```python
from build123d import *

# Parameters (mm, degrees)
SKETCH1_R           = 6.5
BOSS_EXTRUDE1_DEPTH = 1.5
SKETCH2_R           = 5.8
BOSS_EXTRUDE2_DEPTH = 4.3
FILLET1_R           = 0.4
SKETCH3_R           = 5
CUT_EXTRUDE1_DEPTH  = 4.8
BOSS_EXTRUDE3_DEPTH = 4.8
SKETCH5_W           = 2
SKETCH5_H           = 0.8
SKETCH5_W_2         = 1
SKETCH5_H_2         = 3.8
BOSS_EXTRUDE4_DEPTH = 7.2
CUT_EXTRUDE2_REACH  = 10.4
BOSS_EXTRUDE5_DEPTH = 3.8
FILLET2_R           = 0.1
FILLET3_R           = 0.2


with BuildPart() as part:
    # Sketch1 → Boss-Extrude1 (new body)
    with BuildSketch(Plane(origin=(0, 0, 0), x_dir=(1, 0, 0), z_dir=(0, 1, 0))):
        Circle(SKETCH1_R)
    extrude(amount=BOSS_EXTRUDE1_DEPTH)

    # Sketch2 → Boss-Extrude2 (add)
    with BuildSketch(Plane(origin=(0, 1.5, 0), x_dir=(1, 0, 0), z_dir=(0, 1, 0))):
        Circle(SKETCH2_R)
    extrude(amount=BOSS_EXTRUDE2_DEPTH)

    # Fillet1
    fillet1_edges = [part.edges().sort_by_distance(p)[0] for p in [
        (-5.8, 5.8, 0),
    ]]
    fillet(fillet1_edges, radius=FILLET1_R)

    # Sketch3 → Cut-Extrude1 (cut)
    with BuildSketch(Plane.XZ):
        Circle(SKETCH3_R)
    extrude(amount=-CUT_EXTRUDE1_DEPTH, mode=Mode.SUBTRACT)

    # Sketch4 → Boss-Extrude3 (add)
    with BuildSketch(Plane.XZ.offset(-4.8)):
        with BuildLine():
            Line((-4.990991885, 0.3), (-2.9, 0.3))
            Line((-2.9, 0.3), (-2.9, -0.3))
            Line((-2.9, -0.3), (-4.990991885, -0.3))
            ThreePointArc((-4.990991885, -0.3), (-5, 0), (-4.990991885, 0.3))
        make_face()
        with BuildLine():
            Line((2.9, 0.3), (2.9, -0.3))
            Line((2.9, -0.3), (4.990991885, -0.3))
            ThreePointArc((4.990991885, -0.3), (5, 0), (4.990991885, 0.3))
            Line((4.990991885, 0.3), (2.9, 0.3))
        make_face()
        with BuildLine():
            Line((-0.3, 4.990991885), (-0.3, 2.7))
            Line((-0.3, 2.7), (0.3, 2.7))
            Line((0.3, 2.7), (0.3, 4.990991885))
            ThreePointArc((0.3, 4.990991885), (0, 5), (-0.3, 4.990991885))
        make_face()
        with BuildLine():
            Line((0.3, -2.7), (-0.3, -2.7))
            Line((-0.3, -2.7), (-0.3, -4.990991885))
            ThreePointArc((-0.3, -4.990991885), (0, -5), (0.3, -4.990991885))
            Line((0.3, -4.990991885), (0.3, -2.7))
        make_face()
    extrude(amount=BOSS_EXTRUDE3_DEPTH)

    # Sketch5 → Boss-Extrude4 (add)
    with BuildSketch(Plane.XZ.offset(-4.8)):
        with Locations((0, 2.3)):
            Rectangle(SKETCH5_W, SKETCH5_H)
        with Locations((-2.4, 0)):
            Rectangle(SKETCH5_W_2, SKETCH5_H_2)
        with Locations((2.4, 0)):
            Rectangle(SKETCH5_W_2, SKETCH5_H_2)
        with Locations((0, -2.3)):
            Rectangle(SKETCH5_W, SKETCH5_H)
    extrude(amount=BOSS_EXTRUDE4_DEPTH)

    # Sketch6 → Cut-Extrude2 (cut, up to next)
    with BuildSketch(Plane.XY.offset(1.9), mode=Mode.PRIVATE) as cut_extrude2_sk1:
        Polygon((-1.9, -2.4), (-1.9, -1.9625), (-2.4, -2.4), align=None)
    cut_extrude2_tool1 = extrude(cut_extrude2_sk1.sketch, amount=-CUT_EXTRUDE2_REACH, mode=Mode.PRIVATE) & part.part
    add(cut_extrude2_tool1.solids().sort_by_distance((-2.066667, -2.254167, 1.9))[0], mode=Mode.SUBTRACT)
    # Sketch6 → Cut-Extrude2 (cut, up to next)
    with BuildSketch(Plane.XY.offset(1.9), mode=Mode.PRIVATE) as cut_extrude2_sk2:
        Polygon((1.9, -1.9625), (1.9, -2.4), (2.4, -2.4), align=None)
    cut_extrude2_tool2 = extrude(cut_extrude2_sk2.sketch, amount=-CUT_EXTRUDE2_REACH, mode=Mode.PRIVATE) & part.part
    add(cut_extrude2_tool2.solids().sort_by_distance((2.066667, -2.254167, 1.9))[0], mode=Mode.SUBTRACT)

    # Sketch6<3> → Boss-Extrude5 (add)
    with BuildSketch(Plane.XY.offset(1.9)):
        Polygon((-1.6, -1.7), (-1.9, -1.4), (-1.9, -1.9625), align=None)
        Polygon((1.6, -1.7), (1.9, -1.9625), (1.9, -1.4), align=None)
    extrude(amount=-BOSS_EXTRUDE5_DEPTH)

    # Fillet2
    fillet2_edges = [part.edges().sort_by_distance(p)[0] for p in [
        (-1.6, -1.7, 0),
        (1.6, -1.7, 0),
    ]]
    fillet(fillet2_edges, radius=FILLET2_R)

    # Fillet3
    fillet3_edges = [part.edges().sort_by_distance(p)[0] for p in [
        (-6.5, 1.5, 0),
    ]]
    fillet(fillet3_edges, radius=FILLET3_R)


solid = part.part
```
Here's how the part is built. I have some questions about the finished solid (model axes, mm). A direction names the side the tool comes from. Coordinates: 2 decimals unless noted, no trailing zeros. Write each loop counter-clockwise with the first axis right and the second up, starting at its lowest first coordinate (ties: lowest second). Pieces come first, ordered by that corner, then holes. Notation, with made-up numbers: M 54,-6.75 L 64,-6.75 A15 cw 64,-0.75 Z; hole C 10.5,-15.75 d3. An arc over 180 degrees is marked long. Answer as CSV lines item,"result". Start each with the question number.
Q1. If we mould it in two halves opening along X, with no side actions, what happens to faces 1 (the cylindrical face through (-5.794, 3.423, -0.255)), 2 (the flat face through (-2.4, 1.3, -1.9))? For each: pulls with the +X half, pulls with the -X half, needs draft (parallel to the pull), parting line crosses it, or undercut.
Q2. Suppose I cut it at A-A, the plane y = -1. List the corners of the cut face in (x, z) for me, then the cut area to 3 significant figures.
Q3. Will these pins go through, and if not, where does the flat tip stop? pin 1 Ø1.6 at (x, y) = (0.5, 2.5) entering from -Z; pin 2 Ø1 at (y, z) = (0, 2) entering from -X; pin 3 Ø2.5 at (y, z) = (2, 3.5) entering from -X.
Q4. For faces 3 (the flat face through (-1.9, 2, 0)), 4 (the flat face through (2.9, 1.25, -0.45)), which set-ups out of +Z, -Z, +X, -X, +Y, -Y let a thin tool reach every point of the face, with its end or its side?
Q5. I need wall thicknesses on probe 1 along X at (y, z) = (2.5, 1.25); probe 2 along Z at (x, y) = (-0.75, 1); probe 3 along X at (y, z) = (-0.5, -0.5). Which ranges of each line are inside material? Lowest first, please. Write a range as [from, to].
Q6. Suppose I cut it at D-D, the plane z = 0. List the corners of the cut face in (x, y) for me, then the cut area to 3 significant figures.
Q7. Suppose I cut it at C-C, the plane x = 0. List the corners of the cut face in (y, z) for me.
Entries:
1,face 1,"parting line crosses it"
1,face 2,"undercut"
2,outline,"M -2.9,-1.9 L -1.9,-1.9 L -1.9,1.9 L -2.9,1.9 Z; M -1,-2.7 L 1,-2.7 L 1,-1.9 L -1,-1.9 Z; M -1,1.9 L 1,1.9 L 1,2.7 L -1,2.7 Z; M 1.9,-1.9 L 2.9,-1.9 L 2.9,1.9 L 1.9,1.9 Z"
2,area,"10.8 mm²"
3,pin 1,"stops at z = -5.8"
3,pin 2,"stops at x = -6.32"
3,pin 3,"stops at x = -6.02"
4,face 3,"none"
4,face 4,"-Y"
5,probe 1,"x = [-5.66, -4.84], [-2.9, -1.9], [1.9, 2.9], [4.84, 5.66]"
5,probe 2,"z = [-6.46, -4.94], [-2.7, -1.9], [1.9, 2.7], [4.94, 6.46]"
5,probe 3,"x = [-2.9, -1.9], [1.9, 2.9]"
6,outline,"M -6.5,0 L -2.9,0 L -2.9,-2.4 L -2.4,-2.4 L -1.68,-1.77 A0.1 ccw -1.68,-1.62 L -1.9,-1.4 L -1.9,4.8 L 1.9,4.8 L 1.9,-1.4 L 1.68,-1.62 A0.1 ccw 1.68,-1.77 L 2.4,-2.4 L 2.9,-2.4 L 2.9,0 L 6.5,0 L 6.5,1.3 A0.2 ccw 6.3,1.5 L 5.8,1.5 L 5.8,5.4 A0.4 ccw 5.4,5.8 L -5.4,5.8 A0.4 ccw -5.8,5.4 L -5.8,1.5 L -6.3,1.5 A0.2 ccw -6.5,1.3 Z"
6,area,"55.8 mm²"
7,outline,"M -2.4,-2.7 L 0,-2.7 L 0,-6.5 L 1.3,-6.5 A0.2 ccw 1.5,-6.3 L 1.5,-5.8 L 5.4,-5.8 A0.4 ccw 5.8,-5.4 L 5.8,5.4 A0.4 ccw 5.4,5.8 L 1.5,5.8 L 1.5,6.3 A0.2 ccw 1.3,6.5 L 0,6.5 L 0,2.7 L -2.4,2.7 L -2.4,1.9 L 4.8,1.9 L 4.8,-1.9 L -2.4,-1.9 Z"
